The listing builds one solid part. Answer for the finished solid, in the listing's coordinates (mm). A direction names the side the tool comes from. Give positions to 0.01 mm unless a question says otherwise; leave off trailing zeros. Order: outer loops, then holes, each group sorted by start corner. A loop starts at its lowest first (then second) coordinate and runs counter-clockwise, first axis right, second up. Notation, with made-up numbers: (6, 1) - (61, 1) arc R12 ccw to (61, 17) - close; hole circle Ø11 at (8.5, 55.5). An arc over 180 degrees is marked (long way). Answer as a JSON object with one key per item and string values. Group by question number.
Q1. Given pin 1 (6.5 mm diameter, centred on x = 40.5, y = -24.5, fed in from +Z); pin 2 (4 mm diameter, centred on x = 6, y = -1.5, fed in from -Z); pin 3 (4 mm diameter, centred on y = -23.5, z = 15, fed in from -X), each flat-ended and moving along its own axis, determine where each tip first touches the part or whether it passes through.
Q2. The mould has two halves that part along Y. Classify faces 1 (the face through (-38, -36, 12.757)), 2 (the face through (38, -32.512, -7)), 3 (the face through (-38, -25, 23.425)), 4 (the face through (37, -47.752, -6)): released by +Y, released by -Y, zero draft, split by the parting line, or undercut.
Q3. Consider line 1 (X direction, y = -43, z = -7.5); line 2 (Y direction, x = -39, z = 12); line 3 (Z direction, x = 31.5, y = -9). Determine where each line is inside the solid, lowest interval first.
Q4. A cutting plane is placed at B-B, the plane z = -11.5. Give the vertices of the cut face in (x, y).
Q5. A cutting plane is placed at C-C, the plane y = -39. Give the vertices of the cut face in (x, z).
Q6. A cutting plane is placed at D-D, the plane x = 17. Give the vertices of the cut face in (y, z).
Q7. For faces 5 (the face through (31.143, -24, -7)), 6 (the face through (38, -36, -25.343)), 7 (the face through (37, -25, 23.425)), 8 (the face through (-1, -2, 23.586)), determine the directions among +Z, -Z, +X, -X, +Y, -Y from which every point of the face is accessible in a straight line to the end or side of a thin tool.
Q8. A cutting plane is placed at A-A, the plane y = -29. Give the vertices of the cut face in (x, z).
from build123d import *

# Parameters (mm, degrees)
F0_W          = 88.9
F0_H          = 59.69
F1_DEPTH      = 3.81
F2_W          = 12.7
F2_H          = 59.69
F3_DEPTH      = 47.752
F4_W          = 7.62
F4_H          = 38.1
F5_DEPTH      = 25.4
F5_DEPTH_BACK = 25.4
F6_W          = 7.62
F6_H          = 38.1
F7_DEPTH      = 25.4
F7_DEPTH_BACK = 25.4


with BuildPart() as f1:
    # F0 (on Front) → F1 (new body)
    with BuildSketch(Plane.XZ):
        with Locations((-0.312539, -6.258952)):
            Rectangle(F0_W, F0_H)
    extrude(amount=F1_DEPTH)

    # F2 (on Front) → F3 (join)
    with BuildSketch(Plane.XZ):
        with Locations((-38.210436, -6.419758)):
            Rectangle(F2_W, F2_H)
        with Locations((37.492607, -6.419758)):
            Rectangle(F2_W, F2_H)
    extrude(amount=F3_DEPTH)

    # F4 (on face) → F5 (cut, two sides)
    with BuildSketch(Plane.YZ.offset(43.842607)) as f5_sk:
        with Locations((-36.322, -6.292758)):
            Rectangle(F4_W, F4_H)
    extrude(amount=-F5_DEPTH, mode=Mode.SUBTRACT)
    extrude(f5_sk.sketch, amount=-F5_DEPTH_BACK, mode=Mode.SUBTRACT)

    # F6 (on face) → F7 (cut, two sides)
    with BuildSketch(Plane(origin=(-44.560436, 0, 0), x_dir=(0, -1, 0), z_dir=(-1, 0, 0))) as f7_sk:
        with Locations((36.322, -6.292758)):
            Rectangle(F6_W, F6_H)
    extrude(amount=-F7_DEPTH, mode=Mode.SUBTRACT)
    extrude(f7_sk.sketch, amount=-F7_DEPTH_BACK, mode=Mode.SUBTRACT)


solid = f1.part
Reply:
{
 "1": {"pin 1": "stops at z = 23.43", "pin 2": "stops at z = -36.1", "pin 3": "stops at x = -44.56"},
 "2": {"face 1": "undercut", "face 2": "undercut", "face 3": "zero draft", "face 4": "released by -Y"},
 "3": {"line 1": "x = -44.56 to -31.86, 31.14 to 43.84", "line 2": "y = -47.75 to -40.13, -32.51 to 0", "line 3": "z = -36.26 to 23.43"},
 "4": {"outline": "(-44.76, -3.81) - (-44.56, -3.81) - (-44.56, -32.51) - (-31.86, -32.51) - (-31.86, -3.81) - (31.14, -3.81) - (31.14, -32.51) - (43.84, -32.51) - (43.84, -3.81) - (44.14, -3.81) - (44.14, 0) - (-44.76, 0) - close; (-44.56, -47.75) - (-31.86, -47.75) - (-31.86, -40.13) - (-44.56, -40.13) - close; (31.14, -47.75) - (43.84, -47.75) - (43.84, -40.13) - (31.14, -40.13) - close"},
 "5": {"outline": "(-44.56, -36.26) - (-31.86, -36.26) - (-31.86, -25.34) - (-44.56, -25.34) - close; (-44.56, 12.76) - (-31.86, 12.76) - (-31.86, 23.43) - (-44.56, 23.43) - close; (31.14, -36.26) - (43.84, -36.26) - (43.84, -25.34) - (31.14, -25.34) - close; (31.14, 12.76) - (43.84, 12.76) - (43.84, 23.43) - (31.14, 23.43) - close"},
 "6": {"outline": "(-3.81, -36.1) - (0, -36.1) - (0, 23.59) - (-3.81, 23.59) - close"},
 "7": {"face 5": "+Z, -Z, -Y", "face 6": "+X, -X", "face 7": "+Z, +X, -X, -Y", "face 8": "+Z, +X, -X, +Y, -Y"},
 "8": {"outline": "(-44.56, -36.26) - (-31.86, -36.26) - (-31.86, 23.43) - (-44.56, 23.43) - close; (31.14, -36.26) - (43.84, -36.26) - (43.84, 23.43) - (31.14, 23.43) - close"}
}
